The listing builds one solid part. Answer for the finished solid, in the listing's coordinates (mm). Face numbers are marked on the shaded views. A direction names the side the tool comes from. Round coordinates to 2 decimals unless told otherwise and drop trailing zeros. Write each loop counter-clockwise with the first axis right and the second up, starting at its lowest first coordinate (ties: lowest second). Pieces come first, ordered by that corner, then holes.
(1) A cutting plane is placed at C-C, the plane x = 54. Give the vertices of the cut face in (y, z), and give its area (3 significant figures).
(2) The mould has two halves that part along Y. Classify the marked faces 1, 2 and 3: +Y half, -Y half, draft (parallel to the pull), parting line (faces both ways), or undercut.
(3) Each of these flat-tipped pins is pushed along its axis until it touches: pin 1 Ø3 at (x, y) = (-30.31, 567.5) entering from -Z; pin 2 Ø8 at (y, z) = (187.5, 61.5) entering from -X; pin 3 Ø11 at (x, y) = (-17.32, 10) entering from -Z; pin 4 Ø1.5 at (y, z) = (561, 68.5) entering from +X. Where does it stop, or does it pass through?
(4) Find the intervals of material crossed by probe 1 along Y at (x, z) = (0, 82); probe 2 along Y at (x, z) = (-2, 37); probe 3 along X at (y, z) = (567, 85), in increasing order.
(5) For the marked faces 4 and 5, determine the directions among +Z, -Z, +X, -X, +Y, -Y from which every point of the face is accessible in a straight line to the end or side of a thin tool.
(6) A cutting plane is placed at D-D, the plane y = -56. Give the vertices of the cut face in (x, z).
(7) A cutting plane is placed at A-A, the plane y = 612. Give the vertices of the cut face in (x, z).
(8) A cutting plane is placed at B-B, the plane x = -46. Give the vertices of the cut face in (y, z), and give its area (3 significant figures).
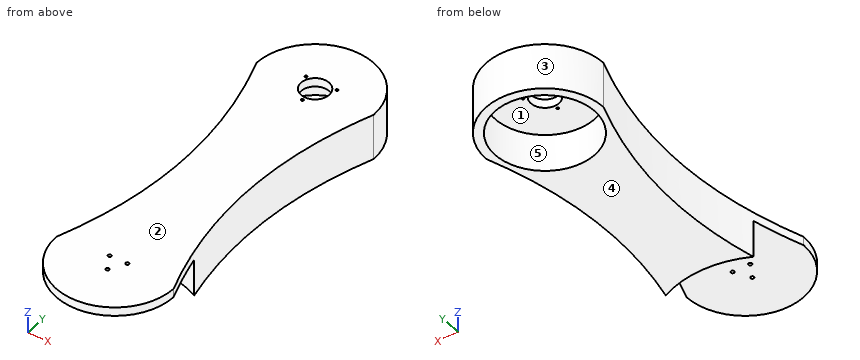
from build123d import *

# Parameters (mm, degrees)
BOSS_EXTRUDE1_DEPTH = 90
SKETCH2_R           = 97.5
CUT_EXTRUDE1_DEPTH  = 72.91
SKETCH6_R           = 97.5
CUT_EXTRUDE5_DEPTH  = 72.91
SKETCH7_R           = 27.5
CUT_EXTRUDE6_DEPTH  = 72.91
CUT_EXTRUDE10_DEPTH = 72.91
SKETCH13_R          = 3.4
CUT_EXTRUDE13_DEPTH = 17.09
SKETCH14_R          = 2.5
CUT_EXTRUDE14_DEPTH = 17.09
CIRPATTERN1_COUNT   = 3


with BuildPart() as part:
    # Sketch1 → Boss-Extrude1 (new body)
    with BuildSketch(Plane(origin=(0, 0, 0), x_dir=(0, 1, 0), z_dir=(0, 0, 1))):
        with BuildLine():
            ThreePointArc((0, 115), (-115, 0), (0, -115))
            add(Edge.make_bspline(
                [(0, -115), (275, -15), (550, -115)],
                knots=[0, 0, 0, 1, 1, 1], degree=2))
            ThreePointArc((550, -115), (665, 0), (550, 115))
            add(Edge.make_bspline(
                [(0, 115), (275, 15), (550, 115)],
                knots=[0, 0, 0, 1, 1, 1], degree=2))
        make_face()
    extrude(amount=BOSS_EXTRUDE1_DEPTH)

    # Sketch2 → Cut-Extrude1 (cut)
    with BuildSketch(Plane(origin=(0, 0, 0), x_dir=(1, 0, 0), z_dir=(0, 0, -1))):
        with Locations(Location((0, 0, 0), (0, 0, 180))):
            Circle(SKETCH2_R)
    extrude(amount=-CUT_EXTRUDE1_DEPTH, mode=Mode.SUBTRACT)

    # Sketch6 → Cut-Extrude5 (cut)
    with BuildSketch(Plane(origin=(0, 0, 0), x_dir=(1, 0, 0), z_dir=(0, 0, -1))):
        with Locations(Location((0, -550, 0), (0, 0, 180))):
            Circle(SKETCH6_R)
    extrude(amount=-CUT_EXTRUDE5_DEPTH, mode=Mode.SUBTRACT)

    # Sketch7 → Cut-Extrude6 (cut)
    with BuildSketch(Plane(origin=(0, 0, 72.91), x_dir=(1, 0, 0), z_dir=(0, 0, -1))):
        with Locations(Location((0, -550, 0), (0, 0, 180))):
            Circle(SKETCH7_R)
    extrude(amount=-CUT_EXTRUDE6_DEPTH, mode=Mode.SUBTRACT)

    # Sketch10 → Cut-Extrude10 (cut)
    with BuildSketch(Plane(origin=(0, 0, 0), x_dir=(1, 0, 0), z_dir=(0, 0, -1))):
        with BuildLine():
            ThreePointArc((115, 0), (0, 115), (-115, 0))
            add(Edge.make_bspline(
                [(-85.785633537, -97.691594321), (-97.237891942, -48.84579716), (-115, 0)],
                knots=[0, 0, 0, 1, 1, 1], degree=2))
            ThreePointArc((-85.785633537, -97.691594321), (0, -117.630315166), (85.785633537, -97.691594321))
            add(Edge.make_bspline(
                [(115, 0), (97.237891942, -48.84579716), (85.785633537, -97.691594321)],
                knots=[0, 0, 0, 1, 1, 1], degree=2))
        make_face()
    extrude(amount=-CUT_EXTRUDE10_DEPTH, mode=Mode.SUBTRACT)

    # Sketch13 → Cut-Extrude13 (cut)
    with BuildSketch(Plane(origin=(0, 0, 72.91), x_dir=(1, 0, 0), z_dir=(0, 0, -1))):
        with Locations(Location((0, 20, 0), (0, 0, 180))):
            Circle(SKETCH13_R)
        with Locations(Location((-17.320508076, -10, 0), (0, 0, 180))):
            Circle(SKETCH13_R)
        with Locations(Location((17.320508076, -10, 0), (0, 0, 180))):
            Circle(SKETCH13_R)
    extrude(amount=-CUT_EXTRUDE13_DEPTH, mode=Mode.SUBTRACT)

    # Sketch14 → Cut-Extrude14 (cut)
    with BuildSketch(Plane.XY.offset(90)):
        with Locations((0, 515)):
            Circle(SKETCH14_R)
    cut_extrude14 = extrude(amount=-CUT_EXTRUDE14_DEPTH, mode=Mode.SUBTRACT)

    # CirPattern1: Cut-Extrude14 ×3 about axis
    cirpattern1_axis = Axis((0, 550, 0), (0, 0, 1))
    for i in range(1, CIRPATTERN1_COUNT):
        add(cut_extrude14.rotate(cirpattern1_axis, i * 360 / CIRPATTERN1_COUNT), mode=Mode.SUBTRACT)


solid = part.part
Solutions:
1. outline: (-101.53, 72.91) - (109.98, 72.91) - (109.98, 0) - (468.82, 0) - (468.82, 72.91) - (631.18, 72.91) - (631.18, 0) - (651.53, 0) - (651.53, 90) - (-101.53, 90) - close
1. area: 40,500 mm2
2. face 1: undercut
2. face 2: draft
2. face 3: +Y half
3. pin 1: passes through
3. pin 2: stops at x = -70.54
3. pin 3: stops at z = 72.91
3. pin 4: stops at x = 114.54
4. probe 1: y = -115 to -23.4, -16.6 to 512.5, 517.5 to 522.5, 577.5 to 665
4. probe 2: y = 117.62 to 452.52, 647.48 to 664.98
4. probe 3: x = -113.74 to -32.76, -27.86 to -21.62, 21.62 to 27.86, 32.76 to 113.74
5. face 4: -Z, +X, -X, +Y, -Y
5. face 5: -Z
6. outline: (-100.44, 72.91) - (100.44, 72.91) - (100.44, 90) - (-100.44, 90) - close
7. outline: (-96.86, 0) - (-75.25, 0) - (-75.25, 72.91) - (75.25, 72.91) - (75.25, 0) - (96.86, 0) - (96.86, 90) - (-96.86, 90) - close
8. outline: (-105.4, 72.91) - (112.11, 72.91) - (112.11, 0) - (464.03, 0) - (464.03, 72.91) - (635.97, 72.91) - (635.97, 0) - (655.4, 0) - (655.4, 90) - (-105.4, 90) - close
8. area: 40,100 mm2
